from build123d import *

# Parameters (mm, degrees)
SKETCH_1_W      = 280
SKETCH_1_H      = 41
SKETCH_1_R      = 6
SKETCH_1_R_2    = 7
SKETCH_1_R_3    = 1.5
SKETCH_1_W_2    = 16
SKETCH_1_H_2    = 14
SKETCH_1_W_3    = 8.5
EXTRUDE_1_DEPTH = 2


with BuildPart() as part:
    # 草图1 → 凸台-拉伸1 (new body)
    with BuildSketch(Plane(origin=(0, 0, 0), x_dir=(1, 0, 0), z_dir=(0, 1, 0))):
        with Locations((140, 20.5)):
            Rectangle(SKETCH_1_W, SKETCH_1_H)
        with Locations((30, 18.7)):
            Circle(SKETCH_1_R, mode=Mode.SUBTRACT)
        with Locations((47, 18.7)):
            Circle(SKETCH_1_R, mode=Mode.SUBTRACT)
        with Locations((64, 18.7)):
            Circle(SKETCH_1_R, mode=Mode.SUBTRACT)
        with Locations((81, 18.7)):
            Circle(SKETCH_1_R, mode=Mode.SUBTRACT)
        with Locations((186.5, 18.7)):
            Circle(SKETCH_1_R_2, mode=Mode.SUBTRACT)
        with Locations((118, 24.7)):
            Circle(SKETCH_1_R_3, mode=Mode.SUBTRACT)
        with Locations((157.5, 18.7)):
            Rectangle(SKETCH_1_W_2, SKETCH_1_H_2, mode=Mode.SUBTRACT)
        with Locations((173.25, 18.7)):
            Rectangle(SKETCH_1_W_3, SKETCH_1_H_2, mode=Mode.SUBTRACT)
    extrude(amount=EXTRUDE_1_DEPTH)


solid = part.part
Can you work these out from the model? Positions are in its coordinate system, mm. Give positions to 0.01 mm unless a question says otherwise; leave off trailing zeros. Write each loop counter-clockwise with the first axis right and the second up, starting at its lowest first coordinate (ties: lowest second). Pieces come first, ordered by that corner, then holes. Notation, with made-up numbers: (-18, 47) -> (24, 47) arc R30 ccw to (24, 86) -> close; hole circle Ø3 at (68.5, -32). An arc over 180 degrees is marked (long way). Answer as a JSON object with one key per item and string values. Group by question number.
Item 1: Suppose I cut it at D-D (x = 27). Please give me the cut outline in (y, z).
Item 2: Please list where these lines run through material, in increasing order: line 1 (Z direction, x = 30, y = 1.5); line 2 (Z direction, x = 186.5, y = 1.4). Write a range as [from, to].
Item 3: Suppose I cut it at A-A (x = 64). Please give me the cut outline in (y, z), plus the area to 3 significant figures.
Item 4: We'd pull the mould along X, two halves only. Please class faces 1 (the face through (59.58, 0.99, -22.76)), 2 (the face through (138, 0, -21)): +X half, -X half, draft (parallel to the pull), parting line (faces both ways), or undercut.
Item 5: I'm going to push a flat-ended pin straight in: P1, Ø7, axis at x = 30, z = -18.7, coming from the -Y side. Where does the tip first touch, or does it pass through?
Item 6: Suppose I cut it at B-B (z = -18.7). State how many separate pieces and enclosed holes the cut face has, plus the area to 3 significant figures.
Findings:
{
 "1": {"outline": "(0, -41) -> (2, -41) -> (2, -23.9) -> (0, -23.9) -> close; (0, -13.5) -> (2, -13.5) -> (2, 0) -> (0, 0) -> close"},
 "2": {"line 1": "z = [-41, -24.7], [-12.7, 0]", "line 2": "z = [-41, -25.7], [-11.7, 0]"},
 "3": {"outline": "(0, -41) -> (2, -41) -> (2, -24.7) -> (0, -24.7) -> close; (0, -12.7) -> (2, -12.7) -> (2, 0) -> (0, 0) -> close", "area": "58.0 mm²"},
 "4": {"face 1": "undercut", "face 2": "draft"},
 "5": {"P1": "passes through"},
 "6": {"separate pieces": "8", "enclosed holes": "0", "area": "387 mm²"}
}
